Read the model definition and answer for the solid it produces. Units are mm, in the model's axes. Give positions to 0.01 mm unless a question says otherwise; leave off trailing zeros. Write each loop counter-clockwise with the first axis right and the second up, starting at its lowest first coordinate (ties: lowest second). Pieces come first, ordered by that corner, then holes. Notation, with made-up numbers: (-30, -14.5) - (2, -14.5) arc R22 ccw to (2, -4.5) - close; hole circle Ø3 at (-21.75, 43). An arc over 180 degrees is marked (long way). Answer as a JSON object with one key per item and string values. Group by question number.
```python
from build123d import *

# Parameters (mm, degrees)
SALIENTE_EXTRUIR1_DEPTH = 1.5
CORTAR_EXTRUIR1_REACH   = 5
CROQUIS2_W              = 3
CROQUIS2_H              = 100


with BuildPart() as part:
    # Croquis1 → Saliente-Extruir1 (new body, symmetric)
    with BuildSketch(Plane(origin=(0, 0, 0), x_dir=(0, 0, -1), z_dir=(1, 0, 0))):
        Polygon((-20, 0), (-15, 0), (-15, -3), (-5, -3), (-5, 0), (5, 0), (5, -3), (15, -3), (15, 0), (20, 0), (20, 200), (15, 200), (15, 203), (5, 203), (5, 200), (-5, 200), (-5, 203), (-15, 203), (-15, 200), (-20, 200), align=None)
    extrude(amount=SALIENTE_EXTRUIR1_DEPTH, both=True)

    # Croquis2 → Cortar-Extruir1 (cut, up to next)
    with BuildSketch(Plane(origin=(1.5, 0, 0), x_dir=(0, 0, -1), z_dir=(1, 0, 0)), mode=Mode.PRIVATE) as cortar_extruir1_sk1:
        with Locations((0, 150)):
            Rectangle(CROQUIS2_W, CROQUIS2_H)
    cortar_extruir1_tool1 = extrude(cortar_extruir1_sk1.sketch, amount=-CORTAR_EXTRUIR1_REACH, mode=Mode.PRIVATE) & part.part
    add(cortar_extruir1_tool1.solids().sort_by_distance((1.5, 150, 0))[0], mode=Mode.SUBTRACT)


solid = part.part
```
1) Flat-ended cylindrical pins translate along their axes: pin 1 Ø0.9 at (x, y) = (-0.5, -1) entering from -Z; pin 2 Ø0.9 at (x, y) = (0, -1.5) entering from +Z; pin 3 Ø0.9 at (x, z) = (0.5, 3) entering from +Y. Find the tip coordinate at first contact, or state that the pin passes through.
2) Find the intervals of material crossed by line 1 (Z direction, x = -1.2, y = 125.5); line 2 (Y direction, x = 0.65, z = -3.5), in increasing order. Write a range as [from, to].
3) Find section B-B, the plane x = 0.95. Write down the section's boundary in (y, z), and give its area (3 significant figures).
4) Find section A-A, the plane y = 115. Write down the section's boundary in (x, z).
Values follow:
{
 "1": {"pin 1": "stops at z = -15", "pin 2": "stops at z = 15", "pin 3": "stops at y = 200"},
 "2": {"line 1": "z = [-20, -1.5], [1.5, 20]", "line 2": "y = [0, 200]"},
 "3": {"outline": "(-3, -15) - (0, -15) - (0, -20) - (200, -20) - (200, -15) - (203, -15) - (203, -5) - (200, -5) - (200, -1.5) - (100, -1.5) - (100, 1.5) - (200, 1.5) - (200, 5) - (203, 5) - (203, 15) - (200, 15) - (200, 20) - (0, 20) - (0, 15) - (-3, 15) - (-3, 5) - (0, 5) - (0, -5) - (-3, -5) - close", "area": "7,820 mm2"},
 "4": {"outline": "(-1.5, -20) - (1.5, -20) - (1.5, -1.5) - (-1.5, -1.5) - close; (-1.5, 1.5) - (1.5, 1.5) - (1.5, 20) - (-1.5, 20) - close"}
}
